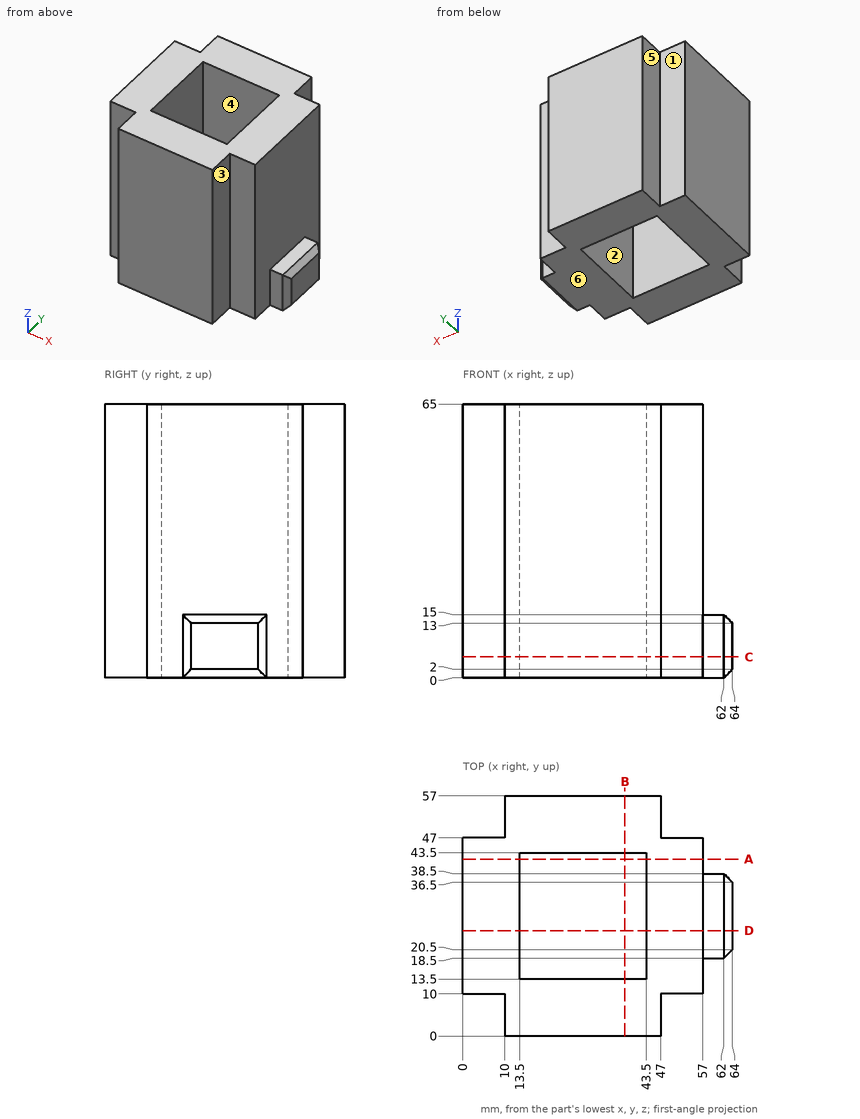
Job drawing, mm, ordinate dimensions from the low corner. One solid piece. A direction names the side the tool comes from. Give positions to 0.01 mm unless a question says otherwise; leave off trailing zeros. Write each loop counter-clockwise with the first axis right and the second up, starting at its lowest first coordinate (ties: lowest second). Pieces come first, ordered by that corner, then holes. Notation, with made-up numbers: M -6.5,-28 L 16.5,-28 A18 ccw 16.5,0 Z; hole C -3.75,11 d1. An arc over 180 degrees is marked long. Put each result on its own line as item: value. Start each with the question number.
(1) Flat gauge pins, fed straight in: pin 1 Ø18.5 at (y, z) = (19.5, 29.5) entering from +X; pin 2 Ø3 at (x, z) = (3, 46.5) entering from -Y; pin 3 Ø5 at (y, z) = (54.5, 18.5) entering from -X. Where does each tip first touch, or does it go through?
(2) Band-saw the part on A-A, the plane y = 42. Write the cut outline in (x, z).
(3) Mould opens along X. For the marked faces 4, 5 and 6 say: +X half, -X half, draft (parallel to the pull), parting line (faces both ways), or undercut.
(4) Band-saw the part on C-C, the plane z = 5. Write the cut outline in (x, y), and give its area (4 significant figures).
(5) Band-saw the part on D-D, the plane y = 25. Write the cut outline in (x, z), and give its area (3 significant figures).
(6) Which spindle directions (+Z, -Z, +X, -X, +Y, -Y) get a long thin tool onto all of the face, cutting with end or side? Do the marked faces 1, 2 and 3. Say none if no direction does.
(7) Probe L1, parallel to X at y = 15, z = 62; L2, parallel to X at y = 4, z = 11. List the from-to ranges inside material, lowest first.
Response values:
1. pin 1: stops at x = 57
1. pin 2: stops at y = 10
1. pin 3: stops at x = 10
2. outline: M 0,0 L 13.5,0 L 13.5,65 L 0,65 Z; M 43.5,0 L 57,0 L 57,65 L 43.5,65 Z
3. face 4: undercut
3. face 5: -X half
3. face 6: draft
4. outline: M 0,10 L 10,10 L 10,0 L 47,0 L 47,10 L 57,10 L 57,18.5 L 62,18.5 L 64,20.5 L 64,36.5 L 62,38.5 L 57,38.5 L 57,47 L 47,47 L 47,57 L 10,57 L 10,47 L 0,47 Z; hole M 13.5,13.5 L 43.5,13.5 L 43.5,43.5 L 13.5,43.5 Z
4. area: 2,085 mm2
5. outline: M 0,0 L 13.5,0 L 13.5,65 L 0,65 Z; M 43.5,0 L 62,0 L 64,2 L 64,13 L 62,15 L 57,15 L 57,65 L 43.5,65 Z
5. area: 1,860 mm2
6. face 1: +Z, -Z, -X, +Y
6. face 2: +Z, -Z
6. face 3: +Z, -Z, +X, -Y
7. L1: x = 0 to 13.5, 43.5 to 57
7. L2: x = 10 to 47
